Source: CAD feature listing. Evaluate the final solid. Frame: model axes, mm. Give positions to 0.01 mm unless a question says otherwise; leave off trailing zeros. Order: outer loops, then holes, each group sorted by start corner. A loop starts at its lowest first (then second) coordinate and runs counter-clockwise, first axis right, second up.
```python
from build123d import *

# Parameters (mm, degrees)
SKETCH1_W                  = 152.4
SKETCH1_H                  = 25.4
EXTRUDE1_DEPTH             = 6.35
F_4_40_TAPPED_HOLE2_D      = 2.2606
F_4_40_TAPPED_HOLE2_DEPTH  = 3.302
F_4_40_TAPPED_HOLE2_TIP    = 0.679152758
F_1_2_0_5_DIAMETER_HOLE1_D = 12.7
F_4_40_TAPPED_HOLE3_D      = 2.2606
F_4_40_TAPPED_HOLE3_DEPTH  = 8.89
F_4_40_TAPPED_HOLE3_TIP    = 0.679152758


with BuildPart() as part:
    # Sketch1 → Extrude1 (new body)
    with BuildSketch(Plane.XY):
        Rectangle(SKETCH1_W, SKETCH1_H)
    extrude(amount=EXTRUDE1_DEPTH)

    # #4-40 Tapped Hole2
    with Locations(Plane(origin=(-69.85, 0, 6.35), x_dir=(1, 0, 0), z_dir=(0, 0, 1))):
        with Locations((0, 0)):
            Hole(F_4_40_TAPPED_HOLE2_D / 2, depth=F_4_40_TAPPED_HOLE2_DEPTH)
            with Locations((0, 0, -(F_4_40_TAPPED_HOLE2_DEPTH + F_4_40_TAPPED_HOLE2_TIP / 2))):  # 118° drill point
                Cone(0, F_4_40_TAPPED_HOLE2_D / 2, F_4_40_TAPPED_HOLE2_TIP, mode=Mode.SUBTRACT)

    # 1/2 (0.5) Diameter Hole1 (through all)
    with Locations(Plane(origin=(25.4, 0, 6.35), x_dir=(1, 0, 0), z_dir=(0, 0, 1))):
        with Locations((0, 0)):
            Hole(F_1_2_0_5_DIAMETER_HOLE1_D / 2)

    # #4-40 Tapped Hole3
    with Locations(Plane(origin=(25.610669662, -12.7, 3.178918451), x_dir=(0, 0, -1), z_dir=(0, -1, 0))):
        with Locations((0, 0)):
            Hole(F_4_40_TAPPED_HOLE3_D / 2, depth=F_4_40_TAPPED_HOLE3_DEPTH)
            with Locations((0, 0, -(F_4_40_TAPPED_HOLE3_DEPTH + F_4_40_TAPPED_HOLE3_TIP / 2))):  # 118° drill point
                Cone(0, F_4_40_TAPPED_HOLE3_D / 2, F_4_40_TAPPED_HOLE3_TIP, mode=Mode.SUBTRACT)

    # Sketch17 → CSK for 1/4 Flat Head Socket Cap Screw4 (revolve, cut)
    with BuildSketch(Plane(origin=(-50.8, 0, 6.35), x_dir=(0, -1, 0), z_dir=(1, 0, 0))):
        Polygon((0, 0), (0, 6.35), (3.3782, 6.35), (3.3782, 3.728390023), (6.61924, 0), align=None)
    revolve(axis=Axis((-50.8, 0, 12.7), (0, 0, -1)), mode=Mode.SUBTRACT)

    # Sketch19 → CSK for 1/4 Flat Head Socket Cap Screw5 (revolve, cut)
    with BuildSketch(Plane(origin=(57.15, 0, 6.35), x_dir=(0, -1, 0), z_dir=(1, 0, 0))):
        Polygon((0, 0), (0, 6.35), (3.3782, 6.35), (3.3782, 3.728390023), (6.61924, 0), align=None)
    revolve(axis=Axis((57.15, 0, 12.7), (0, 0, -1)), mode=Mode.SUBTRACT)


solid = part.part
```
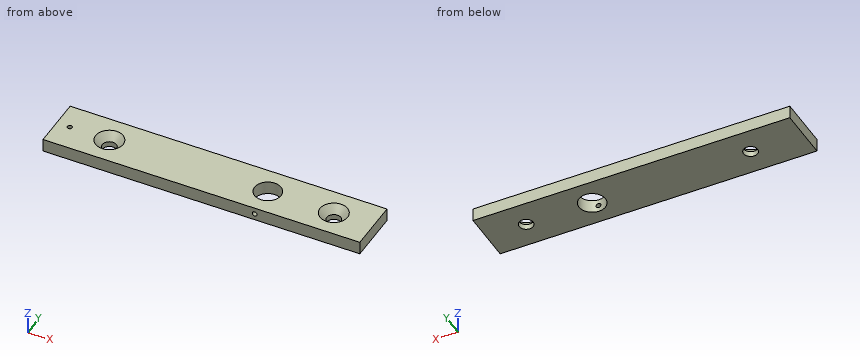
1) Section query A-A, the plane x = 57.15. Return the cut outline in (y, z), and give its area (3 significant figures).
Report:
outline: (-12.7, 0) - (-3.38, 0) - (-3.38, 2.62) - (-6.62, 6.35) - (-12.7, 6.35) - close; (3.38, 0) - (12.7, 0) - (12.7, 6.35) - (6.62, 6.35) - (3.38, 2.62) - close
area: 106 mm2
2) Material intervals for L1, parallel to X at y = -4, z = 4.25; L2, parallel to X at y = -1.75, z = 3.5; L3, parallel to Y at x = -50.8, z = 1.95, sorted ascending.
Report:
L1: x = -76.2 to -53.44, -48.16 to 20.47, 30.33 to 54.51, 59.79 to 76.2
L2: x = -76.2 to -54.55, -47.05 to 19.3, 31.5 to 53.4, 60.9 to 76.2
L3: y = -12.7 to -3.38, 3.38 to 12.7
3) Pin query (flat end, axial travel): pin 1 (11 mm diameter, centred on x = -50.8, y = 0, fed in from +Z); pin 2 (1.8 mm diameter, centred on x = 25.61, z = 3.18, fed in from -Y). Return the tip coordinate at first contact, or that it passes through.
Report:
pin 1: stops at z = 5.06
pin 2: stops at y = 6.25
